Autodesk Inventor part; units mm, degrees
ref_plane "YZ Plane" through (0, 0, 0) normal (1, 0, 0) x (0, 1, 0)
ref_plane "XZ Plane" through (0, 0, 0) normal (0, 1, 0) x (-1, 0, 0)
ref_plane "XY Plane" through (0, 0, 0) normal (0, 0, 1) x (1, 0, 0)
sketch "草图1" plane through (0, 0, 0) normal (0, 0, 1) x (1, 0, 0)
  line L0 (65, -100) -> (-65, -100)
  line L1 (-65, -100) -> (-65, 100)
  line L2 (-65, 100) -> (65, 100)
  line L3 (65, 100) -> (65, -100)
  line L4 (65, -100) -> (-65, 100) construction
  line L5 (-65, -100) -> (65, 100) construction
  point P0 (0, 0)
  dimension "d0" = 130
  dimension "d1" = 200
extrude "拉伸1" add sketch "草图1" along normal blind 3
sketch "草图2" plane through (0, 0, 3) normal (0, 0, 1) x (1, 0, 0)
  line L0 (120, -20) -> (-120, -20)
  line L1 (-120, -20) -> (-120, 20)
  line L2 (-120, 20) -> (120, 20)
  line L3 (120, 20) -> (120, -20)
  line L4 (120, -20) -> (-120, 20) construction
  line L5 (-120, -20) -> (120, 20) construction
  line L6 (-65, 100) -> (-65, -100)
  point P0 (0, 0)
  dimension "d4" = 40
  dimension "d5" = 55
extrude "拉伸2" add sketch "草图2" against normal up to surface (3 mm away)
sketch "草图3" plane through (0, 0, 0) normal (0, 0, -1) x (-1, 0, 0)
  line L0 (120, -20) -> (120, 20)
  line L1 (120, 0) -> (-120, 0)
  line L2 (-120, -20) -> (-120, 20)
  line L3 (71, 49.9947) -> (71, -50.0053)
  line L4 (65, -100) -> (-65, -100)
  line L5 (0, -100) -> (0, 7.1575)
  circle A0 centre (86, -10) radius 2.5
  circle A1 centre (106, -10) radius 2.5
  line L6 (65, -20) -> (120, -20)
  circle A2 centre (86, 10) radius 2.5
  circle A3 centre (106, 10) radius 2.5
  circle A4 centre (-86, -10) radius 2.5
  circle A5 centre (-106, -10) radius 2.5
  circle A6 centre (-86, 10) radius 2.5
  circle A7 centre (-106, 10) radius 2.5
  point P0 (0, 0)
  dimension "d12" = 5
  dimension "d13" = 5
  dimension "d14" = 20
  dimension "d15" = 10
  dimension "d16" = 15
extrude "拉伸3" cut sketch "草图3" against normal blind 10 contours A0 | A1 | A2 | A3 | A4 | A5 | A6 | A7
sketch "草图4" plane through (0, 0, 3) normal (0, 0, 1) x (1, 0, 0)
  line L0 (-30, -90) -> (30, -90)
  line L1 (30, -90) -> (30, -50)
  line L2 (30, -50) -> (-30, -50)
  line L3 (-30, -50) -> (-30, -90)
  line L4 (-30, -90) -> (30, -50) construction
  line L5 (30, -90) -> (-30, -50) construction
  line L6 (-65, -100) -> (65, -100)
  point P0 (0, 0)
  point P1 (0, -70)
  dimension "d17" = 10
  dimension "d18" = 60
  dimension "d19" = 40
extrude "拉伸4" cut sketch "草图4" against normal blind 10
fillet "圆角1" radius 5 4 edges at (30, -90, 1.5) (30, -50, 1.5) (-30, -50, 1.5) (-30, -90, 1.5)
sketch "草图5" plane through (0, 0, 3) normal (0, 0, 1) x (1, 0, 0)
  line L0 (-35, 150) -> (35, 150)
  line L1 (35, 150) -> (35, 50)
  line L2 (35, 50) -> (-35, 50)
  line L3 (-35, 50) -> (-35, 150)
  line L4 (65, 100) -> (-65, 100)
  line L5 (-35, 150) -> (35, 50) construction
  line L6 (35, 150) -> (-35, 50) construction
  point P0 (0, 0)
  point P1 (0, 100)
  dimension "d23" = 50
  dimension "d24" = 70
extrude "拉伸5" cut sketch "草图5" against normal blind 10
fillet "圆角2" radius 5 4 edges at (35, 100, 1.5) (35, 50, 1.5) (-35, 50, 1.5) (-35, 100, 1.5)
sketch "草图6" plane through (0, 0, 3) normal (0, 0, 1) x (1, 0, 0)
  line L0 (-120, -20) -> (-120, 20)
  line L1 (-120, 3) -> (120, 3)
  line L2 (120, -20) -> (120, 20)
  line L3 (-120, 20) -> (-120, -20)
  line L4 (-120, -20) -> (-65, -20)
  line L5 (-51, -94.6609) -> (-51, 98.803)
  line L6 (-65, -20) -> (-65, -100)
  circle A0 centre (-51, 3) radius 2
  point P0 (0, 0)
  dimension "d28" = 23
  dimension "d29" = 14
  dimension "d30" = 4
extrude "拉伸6" cut sketch "草图6" against normal blind 10
ref_plane "工作平面1" through (0, -100, 0) normal (-1, 0, 0) x (0, 0, 1)
mirror "镜像1" about plane through (0, -100, 0) normal (-1, 0, 0) of "拉伸6"
sketch "草图7" plane through (0, 0, 0) normal (0, 0, -1) x (-1, 0, 0)
  line L0 (-8.0092, 31.0916) -> (-13.0092, 31.0916)
  line L1 (-13.0092, 31.0916) -> (-13.0092, 26.0916)
  line L2 (-13.0092, 26.0916) -> (-8.0092, 26.0916)
  line L3 (-8.0092, 26.0916) -> (-8.0092, 31.0916)
  line L4 (-23.0092, 31.0916) -> (-28.0092, 31.0916)
  line L5 (-28.0092, 31.0916) -> (-28.0092, 26.0916)
  line L6 (-28.0092, 26.0916) -> (-23.0092, 26.0916)
  line L7 (-23.0092, 26.0916) -> (-23.0092, 31.0916)
  point P0 (0, 0)
  point P1 (-23.0092, 28.5916)
  point P2 (-13.0092, 28.5916)
  dimension "d33" = 5
  dimension "d34" = 5
  dimension "d35" = 5
  dimension "d36" = 5
  dimension "d37" = 10
extrude "拉伸7" cut sketch "草图7" against normal blind 10
pattern_linear "矩形阵列1" count 2 spacing 50 along (0, -1, 0) of "拉伸7"
sketch "草图8" plane through (0, 0, 0) normal (0, 0, -1) x (-1, 0, 0)
  circle A0 centre (-55, -60) radius 2
  line L0 (65, -100) -> (-65, -100)
  line L1 (-65, -100) -> (-65, -20)
  circle A1 centre (-55, -80) radius 2
  line L2 (-55, -100) -> (-55, -60)
  line L3 (0, 0) -> (-45.6081, 0)
  line L4 (0, 0) -> (0, -68.1904)
  circle A2 centre (55, -60) radius 2
  line L5 (65, -100) -> (65, -20)
  circle A3 centre (55, -80) radius 2
  circle A4 centre (-55, 60) radius 2
  circle A5 centre (-55, 80) radius 2
  circle A6 centre (55, 60) radius 2
  circle A7 centre (55, 80) radius 2
  point P0 (-65, 100)
  point P1 (-55, 100)
  point P2 (0, 68.1904)
  dimension "d43" = 40
  dimension "d45" = 4
  dimension "d46" = 10
  dimension "d47" = 4
  dimension "d48" = 20
extrude "拉伸8" cut sketch "草图8" against normal blind 10
properties part number "板子"
Design review of the part built by this model. Coordinates are the model's own, in mm. A direction names the side the tool comes from. Coordinates: 2 decimals unless noted, no trailing zeros. Write each loop counter-clockwise with the first axis right and the second up, starting at its lowest first coordinate (ties: lowest second). Pieces come first, ordered by that corner, then holes. Notation, with made-up numbers: (-36, -27.75) -> (10, -27.75) arc R22 ccw to (10, -18.75) -> close; hole circle Ø2 at (9.5, 25). An arc over 180 degrees is marked (long way). Write each question's results on one line, items separated by ' | '. Start each with the question number.
(1) Take a section at C-C on y = 10. Write out the cut boundary in (x, z).
(2) Take a section at A-A on x = 86. Write out the cut boundary in (y, z).
(3) Tool access review of faces 1 (the face through (-29, -52, 1)), 2 (the face through (-33, 51, 1)), 3 (the face through (-2, 1, 0)): name each direction out of +Z, -Z, +X, -X, +Y, -Y from which nothing blocks a thin tool from reaching the whole face with its end or side.
(4) The part is to be moulded in two halves that separate along Y. For faces 4 (the face through (34, 52, 1)), 5 (the face through (-2, 1, 3)), 6 (the face through (103.615, -9.249, 1.479)), say which applies: pulls with the +Y half, pulls with the -Y half, needs draft (parallel to the pull), parting line crosses it, or undercut.
(5) Clearance check with flat-ended pins moving along their axes: P1, Ø1.5, axis at y = -55, z = 0.5, coming from the -X side; P2, Ø4.5, axis at x = -106, y = 10, coming from the +Z side; P3, Ø6, axis at x = -106, y = -10, coming from the -Z side; P4, Ø1.5, axis at y = -21.5, z = 1, coming from the +X side. State where each tip first meets the part, or that it passes through.
(6) For line 1 along Y through (x, z) = (-55, 1); line 2 along Y through (x, z) = (-106, 1.25); line 3 along X through (y, z) = (-19.5, 0.9), list the stretches that pass through material, from the lowest coordinate up. Write a range as from..to.
(7) Take a section at D-D on x = -10. Write out the cut boundary in (y, z), and give its area (3 significant figures).
(8) Take a section at B-B on y = 85.5. Write out the cut boundary in (x, z).
Results found:
1) outline: (-120, 0) -> (-108.5, 0) -> (-108.5, 3) -> (-120, 3) -> close; (-103.5, 0) -> (-88.5, 0) -> (-88.5, 3) -> (-103.5, 3) -> close; (-83.5, 0) -> (83.5, 0) -> (83.5, 3) -> (-83.5, 3) -> close; (88.5, 0) -> (103.5, 0) -> (103.5, 3) -> (88.5, 3) -> close; (108.5, 0) -> (120, 0) -> (120, 3) -> (108.5, 3) -> close
2) outline: (-20, 0) -> (-12.5, 0) -> (-12.5, 3) -> (-20, 3) -> close; (-7.5, 0) -> (7.5, 0) -> (7.5, 3) -> (-7.5, 3) -> close; (12.5, 0) -> (20, 0) -> (20, 3) -> (12.5, 3) -> close
3) face 1: +Z, -Z | face 2: +Z, -Z, +Y | face 3: -Z, +X, -X, +Y, -Y
4) face 4: pulls with the +Y half | face 5: needs draft | face 6: undercut
5) P1: stops at x = -65 | P2: passes through | P3: stops at z = 0 | P4: stops at x = 65
6) line 1: y = -100..-82, -78..-62, -58..58, 62..78, 82..100 | line 2: y = -20..-12.5, -7.5..7.5, 12.5..20 | line 3: x = -120..8.01, 13.01..23.01, 28.01..120
7) outline: (-100, 0) -> (-90, 0) -> (-90, 3) -> (-100, 3) -> close; (-50, 0) -> (50, 0) -> (50, 3) -> (-50, 3) -> close | area: 330 mm2
8) outline: (-65, 0) -> (-35, 0) -> (-35, 3) -> (-65, 3) -> close; (35, 0) -> (65, 0) -> (65, 3) -> (35, 3) -> close
